```python
from build123d import *

# Parameters (mm, degrees)
CYLINDER229_R     = 11.2
CYLINDER229_DEPTH = 10
CYLINDER223_R     = 1.7
CYLINDER223_DEPTH = 10
CYLINDER221_R     = 1.4
CYLINDER221_DEPTH = 10
CYLINDER220_R     = 1.7
CYLINDER220_DEPTH = 10
CYLINDER224_R     = 1.7
CYLINDER224_DEPTH = 10
CYLINDER222_R     = 1.7
CYLINDER222_DEPTH = 10
CYLINDER226_R     = 1.4
CYLINDER226_DEPTH = 10
CYLINDER225_R     = 1.4
CYLINDER225_DEPTH = 10
CYLINDER215_R     = 3.1
CYLINDER215_DEPTH = 28
CYLINDER214_R     = 3.1
CYLINDER214_DEPTH = 28
BOX081_W          = 35.6
BOX081_H          = 3
BOX081_DEPTH      = 64


with BuildPart() as cylinder229:
    # Cylinder229 → Cylinder229 (new body)
    with BuildSketch(Plane(origin=(119.7, -14.3, 76.9), x_dir=(1, 0, 0), z_dir=(0, 1, 0))):
        Circle(CYLINDER229_R)
    extrude(amount=CYLINDER229_DEPTH)


with BuildPart() as cylinder223:
    # Cylinder223 → Cylinder223 (new body)
    with BuildSketch(Plane(origin=(135.2, -15, 61.4), x_dir=(1, 0, 0), z_dir=(0, 1, 0))):
        Circle(CYLINDER223_R)
    extrude(amount=CYLINDER223_DEPTH)


with BuildPart() as cylinder221:
    # Cylinder221 → Cylinder221 (new body)
    with BuildSketch(Plane(origin=(120.1, -15, 46.1), x_dir=(1, 0, 0), z_dir=(0, 1, 0))):
        Circle(CYLINDER221_R)
    extrude(amount=CYLINDER221_DEPTH)


with BuildPart() as cylinder220:
    # Cylinder220 → Cylinder220 (new body)
    with BuildSketch(Plane(origin=(104.2, -15, 61.4), x_dir=(1, 0, 0), z_dir=(0, 1, 0))):
        Circle(CYLINDER220_R)
    extrude(amount=CYLINDER220_DEPTH)


with BuildPart() as cylinder224:
    # Cylinder224 → Cylinder224 (new body)
    with BuildSketch(Plane(origin=(104.2, -15, 92.4), x_dir=(1, 0, 0), z_dir=(0, 1, 0))):
        Circle(CYLINDER224_R)
    extrude(amount=CYLINDER224_DEPTH)


with BuildPart() as cylinder222:
    # Cylinder222 → Cylinder222 (new body)
    with BuildSketch(Plane(origin=(135.2, -15, 92.4), x_dir=(1, 0, 0), z_dir=(0, 1, 0))):
        Circle(CYLINDER222_R)
    extrude(amount=CYLINDER222_DEPTH)


with BuildPart() as cylinder226:
    # Cylinder226 → Cylinder226 (new body)
    with BuildSketch(Plane(origin=(135.6, -15, 98.4), x_dir=(1, 0, 0), z_dir=(0, 1, 0))):
        Circle(CYLINDER226_R)
    extrude(amount=CYLINDER226_DEPTH)


with BuildPart() as cylinder225:
    # Cylinder225 → Cylinder225 (new body)
    with BuildSketch(Plane(origin=(104.6, -15, 98.6), x_dir=(1, 0, 0), z_dir=(0, 1, 0))):
        Circle(CYLINDER225_R)
    extrude(amount=CYLINDER225_DEPTH)


with BuildPart() as cylinder215:
    # Cylinder215 → Cylinder215 (new body)
    with BuildSketch(Plane(origin=(129.6, -11.9, 61.3), x_dir=(1, 0, 0), z_dir=(0, 1, 0))):
        Circle(CYLINDER215_R)
    extrude(amount=CYLINDER215_DEPTH)


with BuildPart() as cylinder214:
    # Cylinder214 → Cylinder214 (new body)
    with BuildSketch(Plane(origin=(114, -11.9, 62.4), x_dir=(1, 0, 0), z_dir=(0, 1, 0))):
        Circle(CYLINDER214_R)
    extrude(amount=CYLINDER214_DEPTH)


with BuildPart() as cut269:
    # Box081 → Box081 (new body)
    with BuildSketch(Plane(origin=(102.3, -11, 43.8), x_dir=(1, 0, 0), z_dir=(0, 0, 1))):
        with Locations((17.8, 1.5)):
            Rectangle(BOX081_W, BOX081_H)
    extrude(amount=BOX081_DEPTH)

    # Cut260: cut Cylinder214
    add(cylinder214.part, mode=Mode.SUBTRACT)

    # Cut261: cut Cylinder215
    add(cylinder215.part, mode=Mode.SUBTRACT)

    # Cut262: cut Cylinder225
    add(cylinder225.part, mode=Mode.SUBTRACT)

    # Cut263: cut Cylinder226
    add(cylinder226.part, mode=Mode.SUBTRACT)

    # Cut264: cut Cylinder222
    add(cylinder222.part, mode=Mode.SUBTRACT)

    # Cut265: cut Cylinder224
    add(cylinder224.part, mode=Mode.SUBTRACT)

    # Cut266: cut Cylinder220
    add(cylinder220.part, mode=Mode.SUBTRACT)

    # Cut267: cut Cylinder221
    add(cylinder221.part, mode=Mode.SUBTRACT)

    # Cut268: cut Cylinder223
    add(cylinder223.part, mode=Mode.SUBTRACT)

    # Cut269: cut Cylinder229
    add(cylinder229.part, mode=Mode.SUBTRACT)


solid = cut269.part
```
Could you check a few things on this model? Use its own coordinates, in mm. Round coordinates to 2 decimals unless told otherwise and drop trailing zeros. Loops run counter-clockwise (first coordinate to the right, second up) from the corner with the lowest first, then second, coordinate; pieces in that order, holes last. Notation, with made-up numbers: M 84,15.25 L 128,15.25 A13 ccw 128,39.25 Z; hole C -7.75,26 d3. An arc over 180 degrees is marked long. Put each result on its own line as item: value.
Q1. Imagine slicing it at B-B (y = -10.1). State how many separate pieces and enclosed holes the cut face has, then the cut area to 3 significant figures.
Check result:
separate pieces: 1
enclosed holes: 10
area: 1,770 mm2
Q2. Imagine slicing it at C-C (z = 46.1). Write out the boundary of the cut face in (x, y), then the cut area to 3 significant figures.
Check result:
outline: M 102.3,-11 L 118.7,-11 L 118.7,-8 L 102.3,-8 Z; M 121.5,-11 L 137.9,-11 L 137.9,-8 L 121.5,-8 Z
area: 98.4 mm2
Q3. Imagine slicing it at A-A (x = 113). Write out the boundary of the cut face in (y, z), then the cut area to 3 significant figures.
Check result:
outline: M -11,43.8 L -8,43.8 L -8,59.47 L -11,59.47 Z; M -11,65.33 L -8,65.33 L -8,67.93 L -11,67.93 Z; M -11,85.87 L -8,85.87 L -8,107.8 L -11,107.8 Z
area: 121 mm2
Q4. Thinking about a two-plate mould opening in X: for faces 1 (the face through (136.82, -9.52, 60.89)), 2 (the face through (137.9, -10, 75)), 3 (the face through (120, -9, 107.8)), 4 (the face through (102.3, -10, 75)), which applies, released by +X, released by -X, zero draft, split by the parting line, or undercut?
Check result:
face 1: undercut
face 2: released by +X
face 3: zero draft
face 4: released by -X
Q5. Imagine slicing it at D-D (x = 135.6). Write out the boundary of the cut face in (y, z).
Check result:
outline: M -11,43.8 L -8,43.8 L -8,59.75 L -11,59.75 Z; M -11,63.05 L -8,63.05 L -8,90.75 L -11,90.75 Z; M -11,94.05 L -8,94.05 L -8,97 L -11,97 Z; M -11,99.8 L -8,99.8 L -8,107.8 L -11,107.8 Z
Q6. I need wall thicknesses on probe 1 along Z at (x, y) = (120.1, -10.2); probe 2 along X at (y, z) = (-9.65, 92.4); probe 3 along Z at (x, y) = (135.2, -9.2). Which ranges of each line are inside material? Lowest first, please.
Check result:
probe 1: 43.8 to 44.7, 47.5 to 65.71, 88.09 to 107.8
probe 2: 102.3 to 102.5, 105.9 to 133.5, 136.9 to 137.9
probe 3: 43.8 to 59.7, 63.1 to 90.7, 94.1 to 97.06, 99.74 to 107.8
Q7. For pin 1 (4.5 mm diameter, centred on x = 135.6, z = 98.4, fed in from +Y), with a flat end and sliding along its axis, tell me the tip position at first contact or that it passes through.
Check result:
pin 1: y = -8
